Work out the finished part from the listing and answer in its coordinate system (mm). Coordinates: 2 decimals unless noted, no trailing zeros. Order: outer loops, then holes, each group sorted by start corner. A loop starts at its lowest first (then second) coordinate and runs counter-clockwise, first axis right, second up.
1. Find the intervals of material crossed by probe 1 along X at (y, z) = (0, 8.5); probe 2 along X at (y, z) = (-0.5, 18.5); probe 3 along Y at (x, z) = (-15, -4.5), in increasing order.
2. The part is cut by section B-B, the plane x = 15. Give the vertices of the cut face in (y, z).
3. The part is cut by section C-C, the plane y = 0. Give the vertices of the cut face in (x, z), then the cut area to 3 significant figures.
4. Flat-ended cylindrical pins translate along their axes: pin 1 Ø1.5 at (x, y) = (-15.5, 0.5) entering from +Z; pin 2 Ø2.5 at (x, y) = (14.5, -0.5) entering from +Z. Find the tip coordinate at first contact, or state that the pin passes through.
5. The part is cut by section A-A, the plane z = -12. Give the vertices of the cut face in (x, y), then the cut area to 3 significant figures.
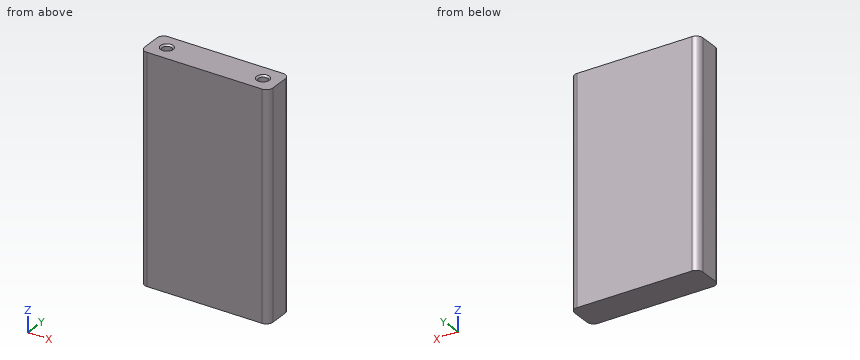
Autodesk Inventor part; units mm, degrees
ref_plane "YZ Plane" through (0, 0, 0) normal (1, 0, 0) x (0, 1, 0)
ref_plane "XZ Plane" through (0, 0, 0) normal (0, 1, 0) x (-1, 0, 0)
ref_plane "XY Plane" through (0, 0, 0) normal (0, 0, 1) x (1, 0, 0)
sketch "Эскиз1" plane through (0, 0, 0) normal (0, 0, 1) x (1, 0, 0)
  line L0 (18, -5) -> (-18, -5)
  line L1 (-20, -3) -> (-20, 3)
  line L2 (-18, 5) -> (18, 5)
  line L3 (20, 3) -> (20, -3)
  line L4 (20, -5) -> (-20, 5) construction
  line L5 (-20, -5) -> (20, 5) construction
  arc A0 (-18, 5) -> (-20, 3) centre (-18, 3) ccw
  arc A1 (-20, -3) -> (-18, -5) centre (-18, -3) ccw
  arc A2 (20, 3) -> (18, 5) centre (18, 3) ccw
  arc A3 (18, -5) -> (20, -3) centre (18, -3) ccw
  point P0 (0, 0)
  dimension "d0" = 40
  dimension "d1" = 10
  dimension "d2" = 2
extrude "Выдавливание1" add sketch "Эскиз1" along normal mid plane 70
sketch "Эскиз2" plane through (0, 0, 35) normal (0, 0, 1) x (1, 0, 0)
  line L0 (0, 0) -> (0, 11.0353) construction
  point P0 (-15, 0)
  point P1 (15, 0)
  dimension "d5" = 30
hole "Отверстие1" at (-15, 0, 35) at (15, 0, 35) direction (0, 0, -1) diameter 3 depth 60
chamfer "Фаска1" distance 0.5 angle 45 2 edges at (-15, 1.5, 35) (15, 1.5, 35)
properties part number "Стенка БСП"
Geometry says:
1. probe 1: x = -20 to -16.5, -13.5 to 13.5, 16.5 to 20
1. probe 2: x = -20 to -16.41, -13.59 to 13.59, 16.41 to 20
1. probe 3: y = -5 to -1.5, 1.5 to 5
2. outline: (-5, -35) - (5, -35) - (5, 35) - (2, 35) - (1.5, 34.5) - (1.5, -25) - (-1.5, -25) - (-1.5, 34.5) - (-2, 35) - (-5, 35) - close
3. outline: (-20, -35) - (20, -35) - (20, 35) - (17, 35) - (16.5, 34.5) - (16.5, -25) - (13.5, -25) - (13.5, 34.5) - (13, 35) - (-13, 35) - (-13.5, 34.5) - (-13.5, -25) - (-16.5, -25) - (-16.5, 34.5) - (-17, 35) - (-20, 35) - close
3. area: 2,440 mm2
4. pin 1: stops at z = -25
4. pin 2: stops at z = 34.96
5. outline: (-20, -3) arc R2 ccw to (-18, -5) - (18, -5) arc R2 ccw to (20, -3) - (20, 3) arc R2 ccw to (18, 5) - (-18, 5) arc R2 ccw to (-20, 3) - close; hole circle Ø3 at (-15, 0); hole circle Ø3 at (15, 0)
5. area: 382 mm2
